Part model, mm, in its own coordinate system. Give positions to 0.01 mm unless a question says otherwise; leave off trailing zeros.
```python
from build123d import *

# Parameters (mm, degrees)
SKETCH1_R           = 2.6035
BOSS_EXTRUDE1_DEPTH = 254


with BuildPart() as part:
    # Sketch1 → Boss-Extrude1 (new body)
    with BuildSketch(Plane(origin=(0, 0, -254), x_dir=(-1, 0, 0), z_dir=(0, 0, -1))):
        with BuildLine():
            Line((12.700000001, -9.550399995), (12.700000001, -6.333083598))
            ThreePointArc((12.700000001, -6.333083598), (12.192000001, -5.825083598), (12.700000001, -5.317083598))
            Line((12.700000001, -5.317083598), (12.700000001, -4.343399998))
            ThreePointArc((12.700000001, -4.343399998), (11.595100001, -3.238499998), (10.490200001, -4.343399998))
            Line((10.490200001, -4.343399998), (10.490200001, -6.474794454))
            ThreePointArc((10.490200001, -6.474794454), (9.863006368, -7.413456059), (8.755779511, -7.193214943))
            Line((8.755779511, -7.193214943), (5.425735971, -3.863171403))
            ThreePointArc((5.425735971, -3.863171403), (4.737482485, -2.83312727), (4.495800001, -1.618107372))
            Line((4.495800001, -1.618107372), (4.495800001, 1.618107372))
            ThreePointArc((4.495800001, 1.618107372), (4.737482485, 2.83312727), (5.425735971, 3.863171403))
            Line((5.425735971, 3.863171403), (8.755779512, 7.193214944))
            ThreePointArc((8.755779512, 7.193214944), (9.863006368, 7.413456059), (10.490200001, 6.474794455))
            Line((10.490200001, 6.474794455), (10.490200001, 4.343399973))
            ThreePointArc((10.490200001, 4.343399973), (11.595100001, 3.238499973), (12.700000001, 4.343399973))
            Line((12.700000001, 4.343399973), (12.700000001, 5.317083602))
            ThreePointArc((12.700000001, 5.317083602), (12.192000001, 5.825083602), (12.700000001, 6.333083602))
            Line((12.700000001, 6.333083602), (12.700000001, 9.550400003))
            ThreePointArc((12.700000001, 9.550400003), (12.192000008, 10.058323495), (12.699846987, 10.566399978))
            ThreePointArc((12.699846987, 10.566399978), (12.082522518, 12.08252252), (10.566399975, 12.699846984))
            ThreePointArc((10.566399975, 12.699846984), (10.058323492, 12.19200001), (9.550400004, 12.700000002))
            Line((9.550400004, 12.700000002), (6.333083601, 12.700000002))
            ThreePointArc((6.333083601, 12.700000002), (5.825083601, 12.192000002), (5.317083601, 12.700000002))
            Line((5.317083601, 12.700000002), (4.343400001, 12.700000002))
            ThreePointArc((4.343400001, 12.700000002), (3.238500001, 11.595100002), (4.343400001, 10.490200002))
            Line((4.343400001, 10.490200002), (6.474794457, 10.490200002))
            ThreePointArc((6.474794457, 10.490200002), (7.413456062, 9.863006369), (7.193214947, 8.755779512))
            Line((7.193214947, 8.755779512), (3.863171407, 5.425735972))
            ThreePointArc((3.863171407, 5.425735972), (2.833127274, 4.737482486), (1.618107376, 4.495800002))
            Line((1.618107376, 4.495800002), (-1.618107374, 4.495800002))
            ThreePointArc((-1.618107374, 4.495800002), (-2.833127271, 4.737482486), (-3.863171404, 5.425735972))
            Line((-3.863171404, 5.425735972), (-7.193214944, 8.755779512))
            ThreePointArc((-7.193214944, 8.755779512), (-7.41345606, 9.863006369), (-6.474794455, 10.490200002))
            Line((-6.474794455, 10.490200002), (-4.34339997, 10.490200002))
            ThreePointArc((-4.34339997, 10.490200002), (-3.23849997, 11.595100002), (-4.34339997, 12.700000002))
            Line((-4.34339997, 12.700000002), (-5.317083599, 12.700000002))
            ThreePointArc((-5.317083599, 12.700000002), (-5.825083599, 12.192000002), (-6.333083599, 12.700000002))
            Line((-6.333083599, 12.700000002), (-9.550399999, 12.700000002))
            ThreePointArc((-9.550399999, 12.700000002), (-10.058323491, 12.192000008), (-10.566399976, 12.699846986))
            ThreePointArc((-10.566399976, 12.699846986), (-12.082522518, 12.082522518), (-12.699846982, 10.566399974))
            ThreePointArc((-12.699846982, 10.566399974), (-12.192000009, 10.058323491), (-12.7, 9.550400003))
            Line((-12.7, 9.550400003), (-12.7, 6.3330836))
            ThreePointArc((-12.7, 6.3330836), (-12.192, 5.8250836), (-12.7, 5.3170836))
            Line((-12.7, 5.3170836), (-12.7, 4.3434))
            ThreePointArc((-12.7, 4.3434), (-11.5951, 3.2385), (-10.4902, 4.3434))
            Line((-10.4902, 4.3434), (-10.4902, 6.474794456))
            ThreePointArc((-10.4902, 6.474794456), (-9.863006367, 7.413456061), (-8.75577951, 7.193214945))
            Line((-8.75577951, 7.193214945), (-5.42573597, 3.863171405))
            ThreePointArc((-5.42573597, 3.863171405), (-4.737482484, 2.833127272), (-4.4958, 1.618107374))
            Line((-4.4958, 1.618107374), (-4.4958, -1.618107374))
            ThreePointArc((-4.4958, -1.618107374), (-4.737482484, -2.833127272), (-5.42573597, -3.863171405))
            Line((-5.42573597, -3.863171405), (-8.75577951, -7.193214945))
            ThreePointArc((-8.75577951, -7.193214945), (-9.863006367, -7.413456061), (-10.4902, -6.474794456))
            Line((-10.4902, -6.474794456), (-10.4902, -4.343399971))
            ThreePointArc((-10.4902, -4.343399971), (-11.5951, -3.238499971), (-12.7, -4.343399971))
            Line((-12.7, -4.343399971), (-12.7, -5.3170836))
            ThreePointArc((-12.7, -5.3170836), (-12.192, -5.8250836), (-12.7, -6.3330836))
            Line((-12.7, -6.3330836), (-12.7, -9.5504))
            ThreePointArc((-12.7, -9.5504), (-12.192000006, -10.058323492), (-12.699846984, -10.566399977))
            ThreePointArc((-12.699846984, -10.566399977), (-12.082522516, -12.082522519), (-10.566399972, -12.699846983))
            ThreePointArc((-10.566399972, -12.699846983), (-10.058323489, -12.192000009), (-9.550400001, -12.700000001))
            Line((-9.550400001, -12.700000001), (-6.333083598, -12.700000001))
            ThreePointArc((-6.333083598, -12.700000001), (-5.825083598, -12.192000001), (-5.317083598, -12.700000001))
            Line((-5.317083598, -12.700000001), (-4.343399998, -12.700000001))
            ThreePointArc((-4.343399998, -12.700000001), (-3.238499998, -11.595100001), (-4.343399998, -10.490200001))
            Line((-4.343399998, -10.490200001), (-6.474794454, -10.490200001))
            ThreePointArc((-6.474794454, -10.490200001), (-7.413456059, -9.863006368), (-7.193214943, -8.755779511))
            Line((-7.193214943, -8.755779511), (-3.863171403, -5.425735971))
            ThreePointArc((-3.863171403, -5.425735971), (-2.83312727, -4.737482485), (-1.618107372, -4.495800001))
            Line((-1.618107372, -4.495800001), (1.618107375, -4.495800001))
            ThreePointArc((1.618107375, -4.495800001), (2.833127273, -4.737482485), (3.863171406, -5.425735971))
            Line((3.863171406, -5.425735971), (7.193214946, -8.755779512))
            ThreePointArc((7.193214946, -8.755779512), (7.413456062, -9.863006368), (6.474794457, -10.490200001))
            Line((6.474794457, -10.490200001), (4.343399973, -10.490200001))
            ThreePointArc((4.343399973, -10.490200001), (3.238499973, -11.595100001), (4.343399973, -12.700000001))
            Line((4.343399973, -12.700000001), (5.317083602, -12.700000001))
            ThreePointArc((5.317083602, -12.700000001), (5.825083602, -12.192000001), (6.333083602, -12.700000001))
            Line((6.333083602, -12.700000001), (9.550400002, -12.700000001))
            ThreePointArc((9.550400002, -12.700000001), (10.058323494, -12.192000007), (10.566399979, -12.699846985))
            ThreePointArc((10.566399979, -12.699846985), (12.082522519, -12.082522518), (12.699846986, -10.566399978))
            ThreePointArc((12.699846986, -10.566399978), (12.192000004, -10.058323491), (12.700000001, -9.550399995))
        make_face()
        with Locations(Location((0, 0, 0), (0, 0, 180))):
            Circle(SKETCH1_R, mode=Mode.SUBTRACT)
    extrude(amount=-BOSS_EXTRUDE1_DEPTH)


solid = part.part
```
1) Two-plate mould, pull along X, no slides. Class faces 1 (the face through (0, 3, 0)), 2 (the face through (2.483, -0.782, -128.778)): +X half, -X half, draft (parallel to the pull), parting line (faces both ways), or undercut.
Answers follow:
face 1: draft
face 2: undercut
2) Wall check: L1, parallel to Y at x = 0, z = -88; L2, parallel to X at y = -4.25, z = -202; L3, parallel to X at y = -5, z = -159. Give the ranges that are in metal, low to high.
Answers follow:
L1: y = -4.5 to -2.6, 2.6 to 4.5
L2: x = -12.7 to -10.49, -5.81 to 5.81, 10.49 to 12.7
L3: x = -12.7 to -10.49, -6.56 to -3.33, 3.33 to 6.56, 10.49 to 12.7
3) Pin check, flat tips, straight feed: pin 1 Ø3.5 at (y, z) = (0.5, -157) entering from +X; pin 2 Ø3 at (x, y) = (2, -9.5) entering from +Z (3 decimals); pin 3 Ø1 at (x, z) = (0, -107) entering from +Y; pin 4 Ø2.5 at (x, z) = (0.5, -185.5) entering from -Y. Stop position of each tip, or through.
Answers follow:
pin 1: stops at x = 4.56
pin 2: passes through
pin 3: stops at y = 4.5
pin 4: stops at y = -4.5
